For this review, take the finished solid that the model builds, in its own axes (mm). Face numbers are marked on the shaded views. A direction names the side the tool comes from. Round coordinates to 2 decimals unless told otherwise and drop trailing zeros. Order: outer loops, then holes, each group sorted by start corner. A loop starts at its lowest first (then second) coordinate and runs counter-clockwise, first axis right, second up. Notation, with made-up numbers: M 30.25,-28 L 87.25,-28 A26 cw 87.25,-9 Z; hole C 88.5,-4.5 d10. An arc over 180 degrees is marked long. Use a Markdown table: item, result.
from build123d import *

# Parameters (mm, degrees)
F1_DEPTH = 22.5
F2_R     = 15
F3_R     = 4
F4_DEPTH = 98.001
F5_R     = 6
F6_DEPTH = 25


with BuildPart() as f1:
    # F0 (on Front) → F1 (new body, symmetric)
    with BuildSketch(Plane.XZ):
        with BuildLine():
            Line((0, 35), (0, 95))
            Line((0, 95), (-5, 95))
            Line((-5, 95), (-5, 35))
            ThreePointArc((-5, 35), (-6.464466, 31.464466), (-10, 30))
            Line((-10, 30), (-20, 30))
            ThreePointArc((-20, 30), (-27.071068, 27.071068), (-30, 20))
            Line((-30, 20), (-30, 10))
            ThreePointArc((-30, 10), (-31.464466, 6.464466), (-35, 5))
            Line((-35, 5), (-98, 5))
            Line((-98, 5), (-98, 0))
            Line((-98, 0), (-35, 0))
            ThreePointArc((-35, 0), (-27.928932, 2.928932), (-25, 10))
            Line((-25, 10), (-25, 20))
            ThreePointArc((-25, 20), (-23.535534, 23.535534), (-20, 25))
            Line((-20, 25), (-10, 25))
            ThreePointArc((-10, 25), (-2.928932, 27.928932), (0, 35))
        make_face()
    extrude(amount=F1_DEPTH, both=True)

    # F2
    f2_edges = [f1.edges().sort_by_distance(p)[0] for p in [
        (-98, -22.5, 2.5),
        (-2.5, -22.5, 95),
        (-2.5, 22.5, 95),
        (-98, 22.5, 2.5),
    ]]
    fillet(f2_edges, radius=F2_R)

    # F3 (on face) → F4 (cut, through all)
    with BuildSketch(Plane.YZ):
        with Locations((0, 85)):
            Circle(F3_R)
    extrude(amount=-F4_DEPTH, mode=Mode.SUBTRACT)

    # F5 (on Top) → F6 (cut)
    with BuildSketch(Plane.XY):
        with Locations((-83, 0)):
            Circle(F5_R)
    extrude(amount=F6_DEPTH, mode=Mode.SUBTRACT)


solid = f1.part
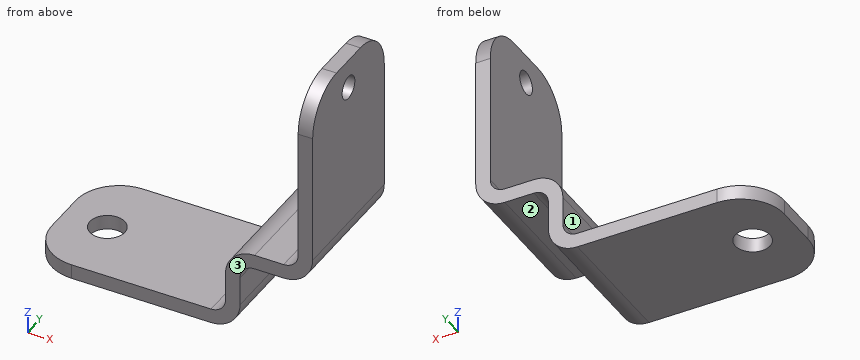
Q1. Add section C-C (y = 9). Write out the cut boundary in (x, z), then the cut area to 3 significant figures.
Determined:
| item | result |
|---|---|
| outline | M -97.92,0 L -35,0 A10 ccw -25,10 L -25,20 A5 cw -20,25 L -10,25 A10 ccw 0,35 L 0,94.92 L -5,94.92 L -5,35 A5 cw -10,30 L -20,30 A10 ccw -30,20 L -30,10 A5 cw -35,5 L -97.92,5 Z |
| area | 891 mm^2 |
Q2. Wall thickness on line 1 along X through (y, z) = (-1.5, 90.5); line 2 along Z through (x, y) = (-47.5, -7); line 3 along X through (y, z) = (0, 1.9): over which ranges is each line inside the solid? List them lowest first. Write a range as [from, to].
Determined:
| item | result |
|---|---|
| line 1 | x = [-5, 0] |
| line 2 | z = [0, 5] |
| line 3 | x = [-98, -89], [-77, -29.14] |
Q3. Add section B-B (z = 85). Write out the cut boundary in (x, y).
Determined:
| item | result |
|---|---|
| outline | M -5,-21.64 L 0,-21.64 L 0,-4 L -5,-4 Z; M -5,4 L 0,4 L 0,21.64 L -5,21.64 Z |
Q4. Add section A-A (y = 0). Write out the cut boundary in (x, z), then the cut area to 3 significant figures.
Determined:
| item | result |
|---|---|
| outline | M -98,0 L -89,0 L -89,5 L -98,5 Z; M -77,0 L -35,0 A10 ccw -25,10 L -25,20 A5 cw -20,25 L -10,25 A10 ccw 0,35 L 0,81 L -5,81 L -5,35 A5 cw -10,30 L -20,30 A10 ccw -30,20 L -30,10 A5 cw -35,5 L -77,5 Z; M -5,89 L 0,89 L 0,95 L -5,95 Z |
| area | 792 mm^2 |
Q5. Clearance check with flat-ended pins moving along their axes: pin 1 (6 mm diameter, centred on x = -75.5, y = 2, fed in from +Z); pin 2 (4 mm diameter, centred on y = -14, z = 27.5, fed in from +X); pin 3 (5 mm diameter, centred on y = -7, z = 13, fed in from -X); pin 4 (7 mm diameter, centred on y = 0, z = 85, fed in from +X). State where each tip first meets the part, or that it passes through.
Determined:
| item | result |
|---|---|
| pin 1 | stops at z = 5 |
| pin 2 | stops at x = -1.65 |
| pin 3 | stops at x = -30 |
| pin 4 | passes through |
Q6. Machinability: for the marked faces 1, 2 and 3, which of the approach directions +Z, -Z, +X, -X, +Y, -Y give a long, thin tool a straight path to every point of the face, cutting with its end or side? Answer none if there is none.
Determined:
| item | result |
|---|---|
| face 1 | +Z, -X, +Y, -Y |
| face 2 | -Z, +X, +Y, -Y |
| face 3 | +Z, -Z, +X, -X, -Y |
Q7. Add section D-D (x = -36.5). Write out the cut boundary in (y, z).
Determined:
| item | result |
|---|---|
| outline | M -22.5,0 L 22.5,0 L 22.5,5 L -22.5,5 Z |
